Here's how the part is built. I have some questions about the finished solid (model axes, mm). A direction names the side the tool comes from. Coordinates: 2 decimals unless noted, no trailing zeros. Write each loop counter-clockwise with the first axis right and the second up, starting at its lowest first coordinate (ties: lowest second). Pieces come first, ordered by that corner, then holes.
from build123d import *

# Parameters (mm, degrees)
SKETCH_2_R               = 2.7
CUT_EXTRUDE_1_DEPTH      = 50.57781762
PATTERN_CIRCULAR_1_COUNT = 3


with BuildPart() as part:
    # 草图1 → 旋转1 (revolve)
    with BuildSketch(Plane.XY, mode=Mode.PRIVATE) as revolve_1_sk:
        Polygon((0, 0), (0, 4.9), (8.2, 4.9), (8.2, 11), (13.2, 11), (13.2, 22), (15.6, 22), (15.6, 11), (51.8, 11), (51.8, 0), align=None)
    revolve(revolve_1_sk.sketch.rotate(Axis((0, 0, 0), (1, 0, 0)), 90), axis=Axis((0, 0, 0), (1, 0, 0)))

    # 草图2 → 切除-拉伸1 (cut, symmetric)
    with BuildSketch(Plane.ZY.offset(-13.2)):
        with Locations((0, 17.5)):
            Circle(SKETCH_2_R)
    cut_extrude_1 = extrude(amount=CUT_EXTRUDE_1_DEPTH, both=True, mode=Mode.SUBTRACT)

    # 阵列(圆周)1: 切除-拉伸1 ×3 about axis
    pattern_circular_1_axis = Axis((0, 0, 0), (1, 0, 0))
    for i in range(1, PATTERN_CIRCULAR_1_COUNT):
        add(cut_extrude_1.rotate(pattern_circular_1_axis, i * 360 / PATTERN_CIRCULAR_1_COUNT), mode=Mode.SUBTRACT)


solid = part.part
1. If I drill on line 1 (Z direction, x = 14, y = -8); line 2 (Y direction, x = 14.65, z = 0); line 3 (Y direction, x = 13, z = 0), over which ranges is the centre line in solid material (lowest first)?
2. Thinking about a two-plate mould opening in Z: for faces 4 (the face through (14.383, 20.177, -0.351)), 5 (the face through (0, 0, 0)), 6 (the face through (4.157, -3.312, -3.612)), which applies, pulls with the +Z half, pulls with the -Z half, needs draft (parallel to the pull), parting line crosses it, or undercut?
3. I want a section at D-D (y = 17.5). List the corners of the cut face in (x, z) for me, then the cut area to 3 significant figures.
4. I want a section at C-C (y = 0). List the corners of the cut face in (x, z) for me, then the cut area to 3 significant figures.
5. I want a section at B-B (y = -8.75). List the corners of the cut face in (x, z) for me.
6. On a 3-axis mill with a long thin cutter (end or side, diameter ignored), from which of +Z, -Z, +X, -X, +Y, -Y can I reach the whole of each face in a straight line? I mean faces 1 (the face through (33.95, 10.74, -2.38)), 2 (the face through (14.417, 21.477, -4.769)), 3 (the face through (10.74, 10.74, -2.38)). Say none if no direction works.
7. For pin 1 Ø2 at (y, z) = (-11.5, 11) entering from -X; pin 2 Ø5 at (x, y) = (12, -10.5) entering from +Z; pin 3 Ø3 at (x, z) = (16.5, -5.5) entering from +Y, each with a flat end and sliding along its axis, tell me the tip position at first contact or that it passes through.
8. I want a section at A-A (z = 0). List the corners of the cut face in (x, y) for me, then the cut area to 3 significant figures.
Response values:
1. line 1: z = -20.49 to -17.75, -12.56 to 12.56, 17.75 to 20.49
1. line 2: y = -22 to 14.8, 20.2 to 22
1. line 3: y = -11 to 11
2. face 4: undercut
2. face 5: needs draft
2. face 6: parting line crosses it
3. outline: (13.2, -13.33) - (15.6, -13.33) - (15.6, -2.7) - (13.2, -2.7) - close; (13.2, 2.7) - (15.6, 2.7) - (15.6, 13.33) - (13.2, 13.33) - close
3. area: 51.0 mm2
4. outline: (0, -4.9) - (8.2, -4.9) - (8.2, -11) - (13.2, -11) - (13.2, -22) - (15.6, -22) - (15.6, -11) - (51.8, -11) - (51.8, 11) - (15.6, 11) - (15.6, 22) - (13.2, 22) - (13.2, 11) - (8.2, 11) - (8.2, 4.9) - (0, 4.9) - close
4. area: 1,090 mm2
5. outline: (8.2, -6.67) - (13.2, -6.67) - (13.2, -12.46) - (15.6, -12.46) - (15.6, -6.67) - (51.8, -6.67) - (51.8, 6.67) - (15.6, 6.67) - (15.6, 12.46) - (13.2, 12.46) - (13.2, 6.67) - (8.2, 6.67) - close; (13.2, -20.19) - (15.6, -20.19) - (15.6, -17.86) - (13.2, -17.86) - close; (13.2, 17.86) - (15.6, 17.86) - (15.6, 20.19) - (13.2, 20.19) - close
6. face 1: +X
6. face 2: +X, -X
6. face 3: -X
7. pin 1: stops at x = 13.2
7. pin 2: stops at z = 20.37
7. pin 3: stops at y = 21.58
8. outline: (0, -4.9) - (8.2, -4.9) - (8.2, -11) - (13.2, -11) - (13.2, -22) - (15.6, -22) - (15.6, -11) - (51.8, -11) - (51.8, 11) - (15.6, 11) - (15.6, 14.8) - (13.2, 14.8) - (13.2, 11) - (8.2, 11) - (8.2, 4.9) - (0, 4.9) - close; (13.2, 20.2) - (15.6, 20.2) - (15.6, 22) - (13.2, 22) - close
8. area: 1,080 mm2
